The drawing under review shows one solid part. Ordinate dimensions are in mm from its lowest x, y, z. A direction names the side the tool comes from. Coordinates: 2 decimals unless noted, no trailing zeros. Order: outer loops, then holes, each group sorted by start corner. A loop starts at its lowest first (then second) coordinate and runs counter-clockwise, first axis right, second up.
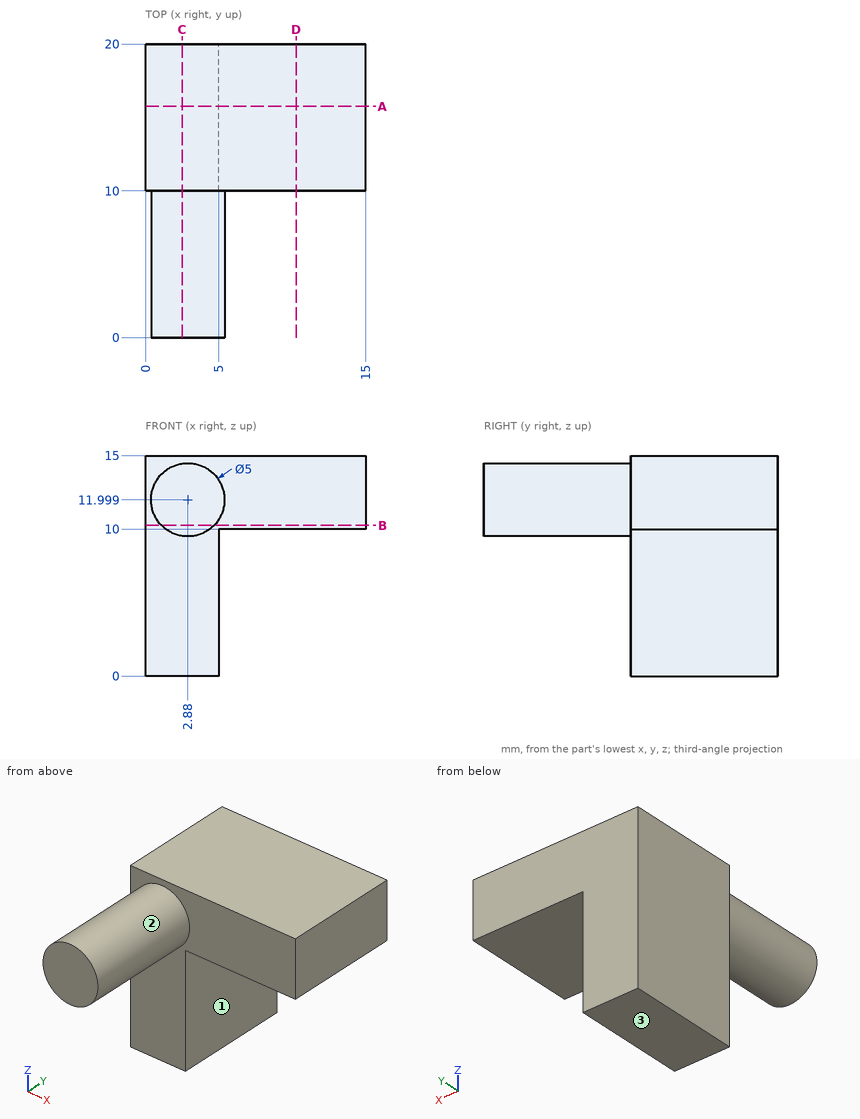
(1) Wall thickness on line 1 (X direction, y = 12.75, z = 6.75); line 2 (Z direction, x = 13.25, y = 15); line 3 (Y direction, x = 4.25, z = 5.5): over which ranges is each line inside the solid? List them lowest first.
(2) Consider section A-A (y = 15.75). Give the boundary of the cut face in (x, z), then the cut area to 3 significant figures.
(3) Consider section D-D (x = 10.25). Give the boundary of the cut face in (y, z).
(4) Consider section B-B (z = 10.25). Give the boundary of the cut face in (x, y), then the cut area to 3 significant figures.
(5) Consider section C-C (x = 2.5). Give the boundary of the cut face in (y, z), then the cut area to 3 significant figures.
(6) Tool access review of the marked faces 1, 2 and 3: name each direction out of +Z, -Z, +X, -X, +Y, -Y from which nothing blocks a thin tool from reaching the whole face with its end or side.
(7) Insertion check: pin 1 Ø7.5 at (x, z) = (6.5, 4.5) entering from -Y; pin 2 Ø5 at (y, z) = (14.5, 3.5) entering from +X; pin 3 Ø2 at (x, y) = (5.5, 3) entering from -Z (1 decimal); pin 4 Ø1.5 at (y, z) = (10.5, 3.5) entering from -X. Each pin has a flat end and moves straight along its axis. Give the tip position at first contact, or say it passes through.
Findings:
1. line 1: x = 0 to 5
1. line 2: z = 10 to 15
1. line 3: y = 10 to 20
2. outline: (0, 0) - (5, 0) - (5, 10) - (15, 10) - (15, 15) - (0, 15) - close
2. area: 125 mm2
3. outline: (10, 10) - (20, 10) - (20, 15) - (10, 15) - close
4. outline: (0, 10) - (1.09, 10) - (1.09, 0) - (4.67, 0) - (4.67, 10) - (15, 10) - (15, 20) - (0, 20) - close
4. area: 186 mm2
5. outline: (0, 9.53) - (10, 9.53) - (10, 0) - (20, 0) - (20, 15) - (10, 15) - (10, 14.47) - (0, 14.47) - close
5. area: 199 mm2
6. face 1: -Z, +X, +Y, -Y
6. face 2: -Y
6. face 3: -Z, +X, -X, +Y, -Y
7. pin 1: stops at y = 10
7. pin 2: stops at x = 5
7. pin 3: stops at z = 10.1
7. pin 4: stops at x = 0
